from build123d import *

# Parameters (mm, degrees)
SKETCH1_R           = 15
BOSS_EXTRUDE1_DEPTH = 104
FILLET1_R           = 15
BOSS_EXTRUDE2_START = 79
SKETCH2_R           = 17
SKETCH2_R_2         = 15
BOSS_EXTRUDE2_DEPTH = 10


with BuildPart() as part:
    # Sketch1 → Boss-Extrude1 (new body)
    with BuildSketch(Plane.XY):
        with Locations(Location((0, 0, 0), (0, 0, 180))):
            Circle(SKETCH1_R)
    extrude(amount=BOSS_EXTRUDE1_DEPTH)

    # Fillet1
    fillet1_edges = [part.edges().sort_by_distance(p)[0] for p in [
        (15, 0, 104),
    ]]
    fillet(fillet1_edges, radius=FILLET1_R)

    # Sketch2 → Boss-Extrude2 (add)
    with BuildSketch(Plane.XY.offset(BOSS_EXTRUDE2_START)):
        Circle(SKETCH2_R)
        with Locations(Location((0, 0, 0), (0, 0, 180))):
            Circle(SKETCH2_R_2, mode=Mode.SUBTRACT)
    extrude(amount=BOSS_EXTRUDE2_DEPTH)


solid = part.part
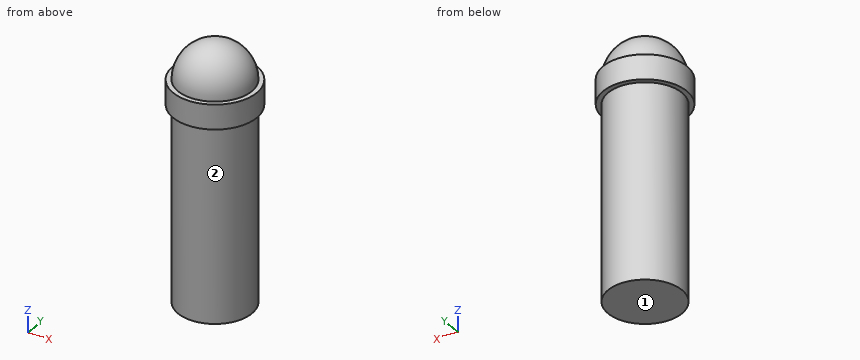
Model file for the job. Use its own axes, mm. Face numbers are marked on the shaded views. A direction names the side the tool comes from. Round coordinates to 2 decimals unless told otherwise and drop trailing zeros. Order: outer loops, then holes, each group sorted by start corner. A loop starts at its lowest first (then second) coordinate and runs counter-clockwise, first axis right, second up.
(1) 3-axis set-ups, long thin cutter, end or side, ignore diameter. For the marked faces 1 and 2: which of +Z, -Z, +X, -X, +Y, -Y reach the whole face in a straight line?
(2) Pin check, flat tips, straight feed: pin 1 (10 mm diameter, centred on x = -5.5, y = 2.5, fed in from -Z); pin 2 (12 mm diameter, centred on y = -4.5, z = 18, fed in from +X); pin 3 (1.5 mm diameter, centred on x = -1, z = 24.5, fed in from +Y); pin 4 (10 mm diameter, centred on x = -4, y = 4.5, fed in from +Z). Stop position of each tip, or through.
(3) Drill centre lines: line 1 (Z direction, x = 13, y = 10.5); line 2 (X direction, y = 7, z = 54.5); line 3 (Z direction, x = 9.5, y = 3). Where is each one in solid material? Low to high.
(4) Band-saw the part on C-C (z = 56). List the corners of the cut face in (x, y), then the cut area to 3 significant figures.
(5) Band-saw the part on A-A (x = 0). List the corners of the cut face in (y, z), then the cut area to 3 significant figures.
Verdict:
1. face 1: -Z, +X, -X, +Y, -Y
1. face 2: -Z
2. pin 1: stops at z = 0
2. pin 2: stops at x = 15
2. pin 3: stops at y = 15
2. pin 4: stops at z = 103.97
3. line 1: z = 79 to 89
3. line 2: x = -13.27 to 13.27
3. line 3: z = 0 to 100.21
4. outline: circle Ø30 at (0, 0)
4. area: 707 mm2
5. outline: (-17, 79) - (-15, 79) - (-15, 0) - (15, 0) - (15, 79) - (17, 79) - (17, 89) - (15, 89) arc R15 ccw to (-15, 89) - (-17, 89) - close
5. area: 3,060 mm2
